Autodesk Inventor part; units mm, degrees
ref_plane "YZ Plane" through (0, 0, 0) normal (1, 0, 0) x (0, 1, 0)
ref_plane "XZ Plane" through (0, 0, 0) normal (0, 1, 0) x (-1, 0, 0)
ref_plane "XY Plane" through (0, 0, 0) normal (0, 0, 1) x (1, 0, 0)
sketch "Sketch1" plane through (0, 0, 0) normal (0, 0, 1) x (1, 0, 0)
  line L0 (-37.8, 0) -> (37.8, 0)
  line L1 (0, -11.2) -> (0, 11.2)
  line L2 (-27, 8) -> (27, 8)
  line L3 (27, 8) -> (27, -8)
  line L4 (27, -8) -> (-27, -8)
  line L5 (-27, -8) -> (-27, 8)
  point P0 (0, 0)
  point P1 (0, 8)
  point P2 (27, 0)
  dimension "d0" = 54
  dimension "d1" = 16
extrude "Extrusion1" add sketch "Sketch1" along normal blind 3
sketch "Sketch2" plane through (0, 0, 3) normal (0, 0, 1) x (1, 0, 0)
  line L0 (-37.8, 0) -> (37.8, 0) construction
  line L1 (0, -11.2) -> (0, 11.2) construction
  point P0 (0, 0)
  point P1 (12, 0)
  dimension "d4" = 12
hole "Hole1" at (12, 0, 3) direction (0, 0, -1) diameter 14.7 end through all
chamfer "Chamfer2" distance 2 angle 45 3 edges at (-27, 8, 1.5) (27, 8, 1.5) (27, -8, 1.5)
chamfer "Chamfer3" distance 4 angle 45 1 edges at (-27, -8, 1.5)
sketch "Sketch3" plane through (0, 0, 3) normal (0, 0, 1) x (1, 0, 0)
  line L0 (-37.8, 0) -> (37.8, 0)
  line L1 (0, -11.2) -> (0, 11.2)
  circle A0 centre (12, 0) radius 7.35
  point P0 (0, 0)
  point P1 (2.47, 0)
  point P2 (21.53, 0)
  dimension "d21" = 9.53
  dimension "d22" = 9.53
hole "Hole2" at (2.47, 0, 3) at (21.53, 0, 3) direction (0, 0, -1) diameter 1.567 end through all
properties part number "P126" material "Aluminium"
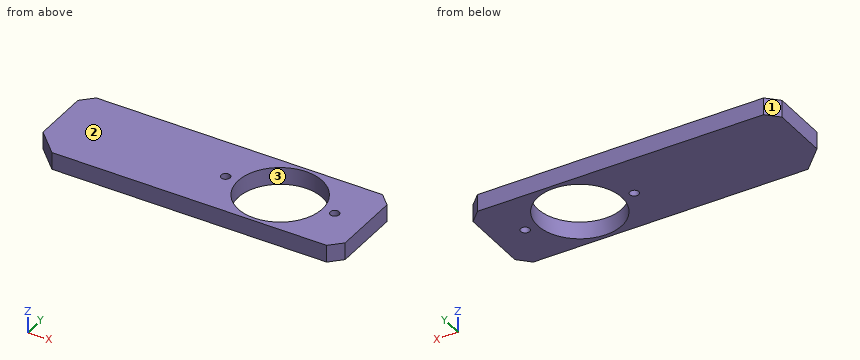
Input: part model. Units: mm. Frame: model coordinates. Face numbers are marked on the shaded views. Coordinates: 2 decimals unless noted, no trailing zeros. Loops run counter-clockwise (first coordinate to the right, second up) from the corner with the lowest first, then second, coordinate; pieces in that order, holes last.
(1) Section B-B on x = 21.53. Return the cut outline in (y, z), then the cut area to 3 significant figures.
(2) Section A-A on y = 0. Return the cut outline in (x, z).
(3) Section D-D on y = 5.25. Return the cut outline in (x, z), then the cut area to 3 significant figures.
(4) Section C-C on z = 0.7. Return the cut outline in (x, y), then the cut area to 3 significant figures.
(5) Material intervals for probe 1 along X at (y, z) = (0, 1.6); probe 2 along Y at (x, z) = (12, 2.2); probe 3 along Y at (x, z) = (21.53, 1.05), sorted ascending.
(6) Pull-direction query (X, two-part tool) for the marked faces 1, 2 and 3; classes: released by +X, released by -X, zero draft, split by the parting line, or undercut.
Data:
1. outline: (-8, 0) - (-0.78, 0) - (-0.78, 3) - (-8, 3) - close; (0.78, 0) - (8, 0) - (8, 3) - (0.78, 3) - close
1. area: 43.3 mm2
2. outline: (-27, 0) - (1.69, 0) - (1.69, 3) - (-27, 3) - close; (3.25, 0) - (4.65, 0) - (4.65, 3) - (3.25, 3) - close; (19.35, 0) - (20.75, 0) - (20.75, 3) - (19.35, 3) - close; (22.31, 0) - (27, 0) - (27, 3) - (22.31, 3) - close
3. outline: (-27, 0) - (6.86, 0) - (6.86, 3) - (-27, 3) - close; (17.14, 0) - (27, 0) - (27, 3) - (17.14, 3) - close
3. area: 131 mm2
4. outline: (-27, -4) - (-23, -8) - (25, -8) - (27, -6) - (27, 6) - (25, 8) - (-25, 8) - (-27, 6) - close; hole circle Ø1.57 at (2.47, 0); hole circle Ø14.7 at (12, 0); hole circle Ø1.57 at (21.53, 0)
4. area: 676 mm2
5. probe 1: x = -27 to 1.69, 3.25 to 4.65, 19.35 to 20.75, 22.31 to 27
5. probe 2: y = -8 to -7.35, 7.35 to 8
5. probe 3: y = -8 to -0.78, 0.78 to 8
6. face 1: released by -X
6. face 2: zero draft
6. face 3: undercut
